Read the model definition and answer for the solid it produces. Units are mm, in the model's axes. Face numbers are marked on the shaded views. A direction names the side the tool comes from. Round coordinates to 2 decimals unless told otherwise and drop trailing zeros. Order: outer loops, then holes, each group sorted by start corner. A loop starts at its lowest first (then second) coordinate and runs counter-clockwise, first axis right, second up. Notation, with made-up numbers: (-16, 28) - (9, 28) arc R21 ccw to (9, 61) - close; hole circle Ø1 at (69, 13). An arc over 180 degrees is marked (long way). Answer as a JSON object with one key per item and string values. Group by question number.
Q1. A cutting plane is placed at D-D on z = 12.5. Count the separate pieces of the cut face and the enclosed holes in it, and give its area (3 significant figures).
Q2. A tool of negligible diameter and unlimited length cuts with its end or side. For the marked faces 4, 5, 6, 7 and 8, from which of +Z, -Z, +X, -X, +Y, -Y can it reach the whole face along a straight path? Write none if from no direction.
Q3. Consider line 1 (Z direction, x = 900, y = 256.5); line 2 (Y direction, x = 900, z = 3.7); line 3 (Z direction, x = 932.5, y = 315.5). Determine where each line is inside the solid, lowest interval first.
Q4. A cutting plane is placed at C-C on z = 3.75. Determine the outline of the cut face in (x, y).
Q5. The mould has two halves that part along X. Classify the marked faces 1, 2 and 3: pulls with the +X half, pulls with the -X half, needs draft (parallel to the pull), parting line crosses it, or undercut.
Q6. A cutting plane is placed at A-A on z = 18.5. Determine the outline of the cut face in (x, y).
Q7. Given pin 1 Ø4 at (x, y) = (890.1, 309.9) entering from +Z; pin 2 Ø4.5 at (x, z) = (900, 12.5) entering from -Y; pin 3 Ø6.5 at (x, z) = (901, 11.5) entering from +Y; pin 4 Ø4 at (x, y) = (880, 261.5) entering from -Z, each flat-ended and moving along its own axis, determine where each tip first touches the part or whether it passes through.
Q8. A cutting plane is placed at B-B on y = 298. Determine the outline of the cut face in (x, z).
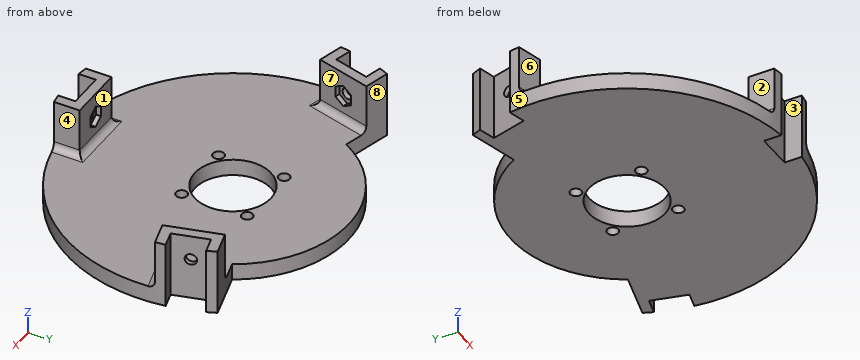
```python
from build123d import *

# Parameters (mm, degrees)
CUT_EXTRUDE_1_DEPTH         = 1013.4351831105043
EXTRUDE_START               = 14.999999999999998
EXTRUDE_1_DEPTH             = 14.999999999999998
CUT_EXTRUDE_2_DEPTH         = 1008.5341185289956
EXTRUDE_2_DEPTH             = 14.999999999999998
CUT_EXTRUDE_3_DEPTH         = 1008.5341185289956
EXTRUDE_3_DEPTH             = 14.999999999999998
CUT_EXTRUDE_4_DEPTH         = 1008.5341185289956
CUT_EXTRUDE_5_DEPTH         = 1.5000000000000013
CUT_EXTRUDE_6_DEPTH         = 1.500000000000375
CUT_EXTRUDE_7_DEPTH         = 1.500000000000482
HOLE_WIZARD_23_0_23_1_D     = 23
HOLE_WIZARD_23_0_23_1_DEPTH = 20
HOLE_WIZARD_3_4_3_4_1_D     = 3.4
HOLE_WIZARD_3_4_3_4_1_DEPTH = 20
HOLE_WIZARD_3_4_3_4_2_D     = 3.4
HOLE_WIZARD_3_4_3_4_2_DEPTH = 6.696579359
HOLE_WIZARD_3_4_3_4_3_D     = 3.4
HOLE_WIZARD_3_4_3_4_3_DEPTH = 14.354957893
HOLE_WIZARD_3_4_3_4_4_D     = 3.4
HOLE_WIZARD_3_4_3_4_4_DEPTH = 14.354957893
FILLET_1_R                  = 2


with BuildPart() as part:
    # 草图1 → 旋转1 (revolve)
    with BuildSketch(Plane.XZ.offset(-300), mode=Mode.PRIVATE) as revolve_1_sk:
        Polygon((950.0000000000001, 5), (900, 4.999999999999999), (900, 0), (950.0000000000001, 0), align=None)
    revolve(revolve_1_sk.sketch.rotate(Axis((900, 300, 4.999999999999999), (0, 0, -1)), 180), axis=Axis((900, 300, 4.999999999999999), (0, 0, -1)))

    # 草图2 → 切除-拉伸1 (cut, through all)
    with BuildSketch(Plane.XY.offset(4.999999999999999)):
        with BuildLine():
            Line((854.6066683745289, 320.9629540842885), (869.404681855504, 316.99783832247647))
            ThreePointArc((869.404681855504, 316.99783832247647), (900, 334.99999999999966), (930.5953181444959, 316.99783832247647))
            Line((930.5953181444959, 316.99783832247647), (945.393331625471, 320.9629540842885))
            ThreePointArc((945.393331625471, 320.9629540842885), (900, 349.9999999999997), (854.6066683745289, 320.9629540842885))
        make_face()
    extrude(amount=-CUT_EXTRUDE_1_DEPTH, mode=Mode.SUBTRACT)

    # 草图3 → 凸台-拉伸1 (add)
    with BuildSketch(Plane.XY.offset(4.999999999999999).offset(EXTRUDE_START)):
        with BuildLine():
            Line((854.6066683745289, 320.9629540842885), (862.114040092375, 318.9513598952115))
            Line((862.114040092375, 318.9513598952115), (857.7141163256321, 302.5306208482976))
            Line((857.7141163256321, 302.5306208482976), (850.206744607786, 304.5422150373745))
            ThreePointArc((850.206744607786, 304.5422150373745), (851.7037086855465, 312.9409522551258), (854.6066683745289, 320.9629540842885))
        make_face()
    extrude(amount=-EXTRUDE_1_DEPTH)

    # 草图4 → 切除-拉伸2 (cut, through all)
    with BuildSketch(Plane.XY.offset(19.999999999999996)):
        with BuildLine():
            Line((850.573285770712, 307.549829170006), (855.592795982073, 306.204855462472))
            Line((855.592795982073, 306.204855462472), (858.4398054782009, 316.830039551652))
            Line((858.4398054782009, 316.830039551652), (853.4202952668401, 318.175013259186))
            ThreePointArc((853.4202952668401, 318.175013259186), (851.7037086855471, 312.9409522551259), (850.573285770712, 307.549829170006))
        make_face()
    extrude(amount=-CUT_EXTRUDE_2_DEPTH, mode=Mode.SUBTRACT)

    # 草图5 → 凸台-拉伸2 (add)
    with BuildSketch(Plane.XY.offset(4.999999999999999).offset(EXTRUDE_START)):
        with BuildLine():
            Line((891.5, 250.7277968830295), (891.5, 258.5))
            Line((891.5, 258.5), (908.5, 258.5))
            Line((908.5, 258.5), (908.5, 250.7277968830295))
            ThreePointArc((908.5, 250.7277968830295), (900, 250.00000000000003), (891.5, 250.7277968830295))
        make_face()
    extrude(amount=-EXTRUDE_2_DEPTH)

    # 草图6 → 切除-拉伸3 (cut, through all)
    with BuildSketch(Plane.XY.offset(19.999999999999996)):
        with BuildLine():
            Line((905.5, 250.30342064085298), (905.5, 255.5))
            Line((905.5, 255.5), (894.5, 255.5))
            Line((894.5, 255.5), (894.5, 250.30342064085298))
            ThreePointArc((894.5, 250.30342064085298), (900, 250.00000000000003), (905.5, 250.30342064085298))
        make_face()
    extrude(amount=-CUT_EXTRUDE_3_DEPTH, mode=Mode.SUBTRACT)

    # 草图7 → 凸台-拉伸3 (add)
    with BuildSketch(Plane.XY.offset(4.999999999999999).offset(EXTRUDE_START)):
        with BuildLine():
            Line((949.7932553922141, 304.5422150373745), (942.285883674368, 302.5306208482975))
            Line((942.285883674368, 302.5306208482975), (937.885959907625, 318.9513598952115))
            Line((937.885959907625, 318.9513598952115), (945.393331625471, 320.9629540842885))
            ThreePointArc((945.393331625471, 320.9629540842885), (948.2962913144532, 312.94095225512575), (949.7932553922141, 304.5422150373745))
        make_face()
    extrude(amount=-EXTRUDE_3_DEPTH)

    # 草图8 → 切除-拉伸4 (cut, through all)
    with BuildSketch(Plane.XY.offset(19.999999999999996)):
        with BuildLine():
            Line((946.5797047331605, 318.17501325918545), (941.5601945218003, 316.83003955165213))
            Line((941.5601945218003, 316.83003955165213), (944.4072040179273, 306.20485546247204))
            Line((944.4072040179273, 306.20485546247204), (949.4267142292881, 307.5498291700056))
            ThreePointArc((949.4267142292881, 307.5498291700056), (948.2962913144534, 312.94095225512547), (946.5797047331605, 318.17501325918545))
        make_face()
    extrude(amount=-CUT_EXTRUDE_4_DEPTH, mode=Mode.SUBTRACT)

    # 草图9 → 切除-拉伸5 (cut)
    with BuildSketch(Plane(origin=(0, 258.5, 0), x_dir=(-1, 0, 0), z_dir=(0, 1, 0))):
        Polygon((-902.857883832489, 14.149999999999999), (-902.857883832489, 10.85), (-900, 9.2), (-897.1421161675111, 10.85), (-897.1421161675121, 14.149999999999999), (-900, 15.8), align=None)
    extrude(amount=-CUT_EXTRUDE_5_DEPTH, mode=Mode.SUBTRACT)

    # 草图10 → 切除-拉伸6 (cut)
    with BuildSketch(Plane(origin=(724.6255099119961, -194.16282019591551, 0), x_dir=(0, 0, -1), z_dir=(0.9659258262890664, -0.25881904510252784, 0))):
        Polygon((-14.149999999999999, 519.8570046465061), (-10.85, 519.8570046465061), (-9.2, 522.7148884789947), (-10.85, 525.5727723114834), (-14.149999999999999, 525.5727723114834), (-15.8, 522.7148884789947), align=None)
    extrude(amount=-CUT_EXTRUDE_6_DEPTH, mode=Mode.SUBTRACT)

    # 草图11 → 切除-拉伸7 (cut)
    with BuildSketch(Plane(origin=(954.7973534939916, 255.83717980410037, 0), x_dir=(0, 0, 1), z_dir=(-0.9659258262890652, -0.2588190451025323, 0))):
        Polygon((10.85, 59.69849112692882), (9.2, 56.8406072944401), (10.85, 53.98272346195163), (14.149999999999999, 53.98272346195163), (15.8, 56.8406072944401), (14.149999999999999, 59.69849112692882), align=None)
    extrude(amount=-CUT_EXTRUDE_7_DEPTH, mode=Mode.SUBTRACT)

    # Ø23.0 (23) 直径孔1
    with Locations(Plane(origin=(0, 0, 0), x_dir=(-1, 0, 0), z_dir=(0, 0, -1))):
        with Locations((-900, 300)):
            Hole(HOLE_WIZARD_23_0_23_1_D / 2, depth=HOLE_WIZARD_23_0_23_1_DEPTH)

    # Ø3.4 (3.4) 直径孔1
    with Locations(Plane(origin=(0, 0, 0), x_dir=(-1, 0, 0), z_dir=(0, 0, -1))):
        with Locations((-909.899494937, 290.100505063), (-909.899494937, 309.899494937), (-890.100505063, 309.899494937), (-890.100505063, 290.100505063)):
            Hole(HOLE_WIZARD_3_4_3_4_1_D / 2, depth=HOLE_WIZARD_3_4_3_4_1_DEPTH)

    # Ø3.4 (3.4) 直径孔2
    with Locations(Plane(origin=(0, 257, 0), x_dir=(1, 0, 0), z_dir=(0, 1, 0))):
        with Locations((900, -12.5)):
            Hole(HOLE_WIZARD_3_4_3_4_2_D / 2, depth=HOLE_WIZARD_3_4_3_4_2_DEPTH)

    # Ø3.4 (3.4) 直径孔3
    with Locations(Plane(origin=(723.1766211725698, -193.77459162825534, 0), x_dir=(0, 0, -1), z_dir=(0.9659258262890692, -0.2588190451025174, 0))):
        with Locations((-12.5, 522.714888479)):
            Hole(HOLE_WIZARD_3_4_3_4_3_D / 2, depth=HOLE_WIZARD_3_4_3_4_3_DEPTH)

    # Ø3.4 (3.4) 直径孔4
    with Locations(Plane(origin=(956.2462422334311, 256.22540837172977, 0), x_dir=(0, 0, 1), z_dir=(-0.9659258262890719, -0.25881904510250775, 0))):
        with Locations((12.5, 56.840607294)):
            Hole(HOLE_WIZARD_3_4_3_4_4_D / 2, depth=HOLE_WIZARD_3_4_3_4_4_DEPTH)

    # 圆角1
    fillet_1_edges = [part.edges().sort_by_distance(p)[0] for p in [
        (853.9604304667091, 303.536417942836, 4.999999999999999),
        (859.9140782090035, 310.74099037175455, 4.999999999999999),
        (908.5, 254.61389844151475, 4.999999999999999),
        (900, 258.5, 4.999999999999999),
        (891.5, 254.61389844151475, 4.999999999999999),
        (940.0859217909965, 310.7409903717545, 4.999999999999999),
        (946.0395695332911, 303.536417942836, 4.999999999999999),
    ]]
    fillet(fillet_1_edges, radius=FILLET_1_R)


solid = part.part
```
Result set:
{
 "1": {"separate pieces": "6", "enclosed holes": "0", "area": "202 mm²"},
 "2": {"face 4": "+Z, +X, +Y, -Y", "face 5": "+Z, -Z, -X", "face 6": "+Z, -X, -Y", "face 7": "+Z, -Y", "face 8": "+Z, -Z, +Y"},
 "3": {"line 1": "z = 0 to 10.8, 14.2 to 20", "line 2": "y = 255.5 to 288.5, 311.5 to 335", "line 3": "z = 0 to 5"},
 "4": {"outline": "(850.57, 307.55) arc R50 ccw to (894.5, 250.3) - (894.5, 255.5) - (905.5, 255.5) - (905.5, 250.3) arc R50 ccw to (949.43, 307.55) - (944.41, 306.2) - (941.56, 316.83) - (946.58, 318.18) arc R50 ccw to (945.39, 320.96) - (930.6, 317) arc R35 ccw to (869.4, 317) - (854.61, 320.96) arc R50 ccw to (853.42, 318.18) - (858.44, 316.83) - (855.59, 306.2) - close; hole circle Ø3.4 at (890.1, 290.1); hole circle Ø3.4 at (890.1, 309.9); hole circle Ø23 at (900, 300); hole circle Ø3.4 at (909.9, 290.1); hole circle Ø3.4 at (909.9, 309.9)"},
 "5": {"face 1": "needs draft", "face 2": "pulls with the -X half", "face 3": "undercut"},
 "6": {"outline": "(850.21, 304.54) - (857.71, 302.53) - (862.11, 318.95) - (854.61, 320.96) arc R50 ccw to (853.42, 318.18) - (858.44, 316.83) - (855.59, 306.2) - (850.57, 307.55) arc R50 ccw to start; (891.5, 250.73) arc R50 ccw to (894.5, 250.3) - (894.5, 255.5) - (905.5, 255.5) - (905.5, 250.3) arc R50 ccw to (908.5, 250.73) - (908.5, 258.5) - (891.5, 258.5) - close; (937.89, 318.95) - (942.29, 302.53) - (949.79, 304.54) arc R50 ccw to (949.43, 307.55) - (944.41, 306.2) - (941.56, 316.83) - (946.58, 318.18) arc R50 ccw to (945.39, 320.96) - close"},
 "7": {"pin 1": "stops at z = 5", "pin 2": "stops at y = 255.5", "pin 3": "stops at y = 258.5", "pin 4": "stops at z = 0"},
 "8": {"outline": "(850.04, 0) - (888.68, 0) - (888.68, 5) - (850.04, 5) - close; (911.32, 0) - (949.96, 0) - (949.96, 5) - (911.32, 5) - close"}
}
